```python
from build123d import *

# Parameters (mm, degrees)
F3_DEPTH      = 12.701
F3_DEPTH_BACK = 12.701


with BuildPart() as f1:
    # F0 (on Front) → F1 (revolve)
    with BuildSketch(Plane.XZ):
        Polygon((0, -20.6375), (0, 20.6375), (-7.9375, 20.6375), (-7.9375, 1.5875), (-12.7, 1.5875), (-12.7, -4.7625), (-10.31875, -4.7625), (-10.31875, -14.2875), (-12.7, -14.2875), (-12.7, -20.6375), align=None)
    revolve(axis=Axis((0, 0, 0), (0, 0, -1)))

    # F2 (on Front) → F3 (cut, two sides)
    with BuildSketch(Plane.XZ) as f3_sk:
        with BuildLine():
            ThreePointArc((0, 13.096875), (-1.403165, 9.709335), (1.984375, 11.1125))
            ThreePointArc((1.984375, 11.1125), (1.403165, 12.515665), (0, 13.096875))
        make_face()
    extrude(amount=F3_DEPTH, mode=Mode.SUBTRACT)
    extrude(f3_sk.sketch, amount=-F3_DEPTH_BACK, mode=Mode.SUBTRACT)


solid = f1.part
```
Model file for the job. Use its own axes, mm. A direction names the side the tool comes from. Coordinates: 2 decimals unless noted, no trailing zeros. Order: outer loops, then holes, each group sorted by start corner. A loop starts at its lowest first (then second) coordinate and runs counter-clockwise, first axis right, second up. Notation, with made-up numbers: (64, 3.5) - (78, 3.5) arc R13 ccw to (78, 28.5) - close; hole circle Ø7 at (74, 84). An arc over 180 degrees is marked (long way). Return JSON: item names as keys, results as strings. Group by question number.
1) Saw through at C-C, the plane z = 12. Write the cut outline in (x, y) (1 decimal), plus the area to 3 significant figures.
2) Probe line 1 (Z direction, x = 3, y = -10.25); line 2 (Z direction, x = 0, y = 4.5); line 3 (Z direction, x = -9.25, y = 2.5). List the from-to ranges inside material, lowest first. Write a range as from..to.
3) Saw through at A-A, the plane y = 0. Write the cut outline in (x, z).
4) Saw through at B-B, the plane x = 1.5. Write the cut outline in (y, z).
5) Flat gauge pins, fed straight in: P1, Ø1.5, axis at x = -3.5, z = -9, coming from the +Y side; P2, Ø8, axis at x = -9, z = 9.5, coming from the +Y side; P3, Ø1, axis at y = -7.5, z = 7.5, coming from the -X side; P4, Ø2.5, axis at x = 0, z = 11.11, coming from the -Y side. Where does each tip first touch, or does it go through?
6) Tool access for faces 1 (the flat face through (-1.9, 10.4, -14.288)), 2 (the cylindrical face through (-7.332, -3.04, 10.979)), 3 (the flat face through (0, 0, 20.638)): list every direction of +Z, -Z, +X, -X, +Y, -Y with a clear straight run to the whole face (end or side of a thin tool).
7) Saw through at D-D, the plane y = 5.75. Write the cut outline in (x, z), plus the area to 3 significant figures.
8) Mould opens along Z. For faces 4 (the cylindrical face through (2.237, -10.073, -9.592)), 5 (the flat face through (-0.2, -8.3, 1.588)), 6 (the flat face through (0, 0, -20.638)) say: released by +Z, released by -Z, zero draft, split by the parting line, or undercut.
Values found:
{
 "1": {"outline": "(-1.8, -7.7) - (-1.8, 7.7) arc R7.9 ccw to start; (1.8, -7.7) arc R7.9 ccw to (1.8, 7.7) - close", "area": "142 mm²"},
 "2": {"line 1": "z = -20.64..-14.29, -4.76..1.59", "line 2": "z = -20.64..9.13, 13.1..20.64", "line 3": "z = -20.64..1.59"},
 "3": {"outline": "(-12.7, -20.64) - (12.7, -20.64) - (12.7, -14.29) - (10.32, -14.29) - (10.32, -4.76) - (12.7, -4.76) - (12.7, 1.59) - (7.94, 1.59) - (7.94, 20.64) - (-7.94, 20.64) - (-7.94, 1.59) - (-12.7, 1.59) - (-12.7, -4.76) - (-10.32, -4.76) - (-10.32, -14.29) - (-12.7, -14.29) - close; hole circle Ø3.97 at (0, 11.11)"},
 "4": {"outline": "(-12.61, -20.64) - (12.61, -20.64) - (12.61, -14.29) - (10.21, -14.29) - (10.21, -4.76) - (12.61, -4.76) - (12.61, 1.59) - (7.79, 1.59) - (7.79, 9.81) - (-7.79, 9.81) - (-7.79, 1.59) - (-12.61, 1.59) - (-12.61, -4.76) - (-10.21, -4.76) - (-10.21, -14.29) - (-12.61, -14.29) - close; (-7.79, 12.41) - (7.79, 12.41) - (7.79, 20.64) - (-7.79, 20.64) - close"},
 "5": {"P1": "stops at y = 9.95", "P2": "stops at y = 6.16", "P3": "stops at x = -3.74", "P4": "passes through"},
 "6": {"face 1": "none", "face 2": "+Z", "face 3": "+Z, +X, -X, +Y, -Y"},
 "7": {"outline": "(-11.32, -20.64) - (11.32, -20.64) - (11.32, -14.29) - (8.57, -14.29) - (8.57, -4.76) - (11.32, -4.76) - (11.32, 1.59) - (5.47, 1.59) - (5.47, 20.64) - (-5.47, 20.64) - (-5.47, 1.59) - (-11.32, 1.59) - (-11.32, -4.76) - (-8.57, -4.76) - (-8.57, -14.29) - (-11.32, -14.29) - close; hole circle Ø3.97 at (0, 11.11)", "area": "647 mm²"},
 "8": {"face 4": "undercut", "face 5": "released by +Z", "face 6": "released by -Z"}
}
